Autodesk Inventor part; units mm, degrees
ref_plane "YZ Plane" through (0, 0, 0) normal (1, 0, 0) x (0, 1, 0)
ref_plane "XZ Plane" through (0, 0, 0) normal (0, 1, 0) x (-1, 0, 0)
ref_plane "XY Plane" through (0, 0, 0) normal (0, 0, 1) x (1, 0, 0)
sketch "Skizze1" plane through (0, 0, 0) normal (0, 0, 1) x (1, 0, 0)
  line L0 (-6.5297, -2.8796) -> (43.4703, -2.8796)
  line L1 (43.4703, -2.8796) -> (43.4703, 8.1204)
  line L2 (43.4703, 8.1204) -> (-6.5297, 8.1204)
  line L3 (-6.5297, 8.1204) -> (-6.5297, -2.8796)
  point P0 (0, 0)
  dimension "d0" = 50
  dimension "d1" = 11
extrude "Extrusion1" add sketch "Skizze1" along normal blind 7
sketch "Skizze2" plane through (-6.5297, 8.1204, 0) normal (0, 1, 0) x (1, 0, 0)
  line L0 (29.65, -5.55) -> (20.35, -5.55)
  line L1 (20.35, -5.55) -> (20.35, -1.45)
  line L2 (20.35, -1.45) -> (29.65, -1.45)
  line L3 (29.65, -1.45) -> (29.65, -5.55)
  line L4 (50, -7) -> (0, -7)
  line L5 (50, 0) -> (50, -7)
  line L6 (0, 0) -> (0, -7)
  point P0 (6.5297, 0)
  dimension "d4" = 9.3
  dimension "d5" = 4.1
  dimension "d6" = 1.45
  dimension "d7" = 20.35
  dimension "d8" = 20.35
extrude "Extrusion2" cut sketch "Skizze2" against normal blind 8.35
sketch "Skizze3" plane through (0, 0, 7) normal (0, 0, 1) x (1, 0, 0)
  line L0 (-6.5297, 8.1204) -> (-6.5297, -2.8796)
  line L1 (43.4703, 8.1204) -> (-6.5297, 8.1204)
  point P0 (0, 0)
  point P1 (5.9703, 2.2704)
  point P2 (18.4703, 2.2704)
  point P3 (30.9703, 2.2704)
  dimension "d11" = 12.5
  dimension "d12" = 12.5
  dimension "d13" = 12.5
  dimension "d14" = 5.85
hole "Bohrung1" at (5.9703, 2.2704, 7) at (18.4703, 2.2704, 7) at (30.9703, 2.2704, 7) direction (0, 0, -1) diameter 6.15 end through all
sketch "Skizze4" plane through (-6.5297, 8.1204, 0) normal (0, 1, 0) x (1, 0, 0)
  point P0 (6.5297, 0)
sketch "Skizze5" plane through (-6.5297, 8.1204, 0) normal (0, 1, 0) x (1, 0, 0)
  line L0 (50, 0) -> (0, 0)
  line L1 (0, 0) -> (0, -53.0037)
  line L2 (0, -53) -> (50, -53)
  line L3 (50, -53) -> (50, 46)
  line L4 (50, 46) -> (0, 46)
  line L5 (0, 46) -> (0, -53)
  point P0 (6.5297, 0)
  dimension "d22" = 50
  dimension "d23" = 99
  dimension "d24" = 46
extrude "Extrusion3" add sketch "Skizze5" along normal blind 3.5
sketch "Skizze6" plane through (-6.5297, 11.6204, 0) normal (0, 1, 0) x (1, 0, 0)
  line L0 (29.65, -1.45) -> (29.65, -5.55)
  line L1 (29.65, -1.45) -> (20.35, -1.45)
  line L2 (20.35, -1.45) -> (20.35, -5.55)
  line L3 (20.35, -5.55) -> (29.65, -5.55)
  line L4 (29.65, -5.55) -> (29.65, -1.45)
  point P0 (6.5297, 0)
extrude "Extrusion4" cut sketch "Skizze6" against normal blind 3.5
sketch "Skizze7" plane through (-6.5297, 11.6204, 0) normal (0, 1, 0) x (1, 0, 0)
  line L0 (0, -53) -> (50, -53)
  line L1 (50, -53) -> (42.5, -53)
  line L2 (42.5, -53) -> (42.5, -42.5)
  line L3 (42.5, -42.5) -> (50, -42.5)
  line L4 (50, -42.5) -> (50, -53)
  line L5 (0, -53) -> (7.5, -53)
  line L6 (7.5, -53) -> (7.5, -42.5)
  line L7 (7.5, -42.5) -> (0, -42.5)
  line L8 (0, -42.5) -> (0, -53)
  line L9 (0, 46) -> (0, -53)
  line L10 (0, 46) -> (7.5, 46)
  line L11 (7.5, 46) -> (7.5, 35.5)
  line L12 (7.5, 35.5) -> (0, 35.5)
  line L13 (0, 35.5) -> (0, 46)
  line L14 (50, -53) -> (50, 46)
  line L15 (50, 46) -> (42.5, 46)
  line L16 (42.5, 46) -> (42.5, 35.5)
  line L17 (42.5, 35.5) -> (50, 35.5)
  line L18 (50, 35.5) -> (50, 46)
  point P0 (6.5297, 0)
  dimension "d29" = 7.5
  dimension "d30" = 10.5
  dimension "d31" = 7.5
  dimension "d32" = 10.5
  dimension "d33" = 7.5
  dimension "d34" = 10.5
  dimension "d35" = 7.5
  dimension "d36" = 10.5
extrude "Extrusion5" add sketch "Skizze7" along normal blind 25
sketch "Skizze8" plane through (0.9703, 11.6204, -35.5) normal (1, 0, 0) x (0, 0, -1)
  point P0 (-35.5, -11.6204)
sketch "Skizze9" plane through (-6.5297, 36.6204, 0) normal (0, 1, 0) x (1, 0, 0)
  line L0 (50, -42.5) -> (50, 35.5)
  line L1 (0, 46) -> (50, 46)
  line L2 (50, 46) -> (50, 35.5)
  line L3 (50, 35.5) -> (0, 35.5)
  line L4 (0, 35.5) -> (0, 46)
  line L5 (50, -53) -> (50, -7)
  line L6 (0, -42.5) -> (50, -42.5)
  line L7 (50, -42.5) -> (50, -53)
  line L8 (50, -53) -> (0, -53)
  line L9 (0, -53) -> (0, -42.5)
  line L10 (50, -42.5) -> (42.5, -42.5)
  point P0 (6.5297, 0)
  dimension "d75" = 0
extrude "Extrusion6" add sketch "Skizze9" along normal blind 5
sketch "Skizze10" plane through (-6.5297, 41.6204, 0) normal (0, 1, 0) x (1, 0, 0)
  line L0 (50, 46) -> (0, 46)
  line L1 (0, -53) -> (50, -53)
  line L2 (42.5, -42.5) -> (42.5, -53)
  line L3 (42.5, 46) -> (42.5, 35.5)
  line L4 (7.5, 35.5) -> (7.5, 46)
  line L5 (7.5, -53) -> (7.5, -42.5)
  point P0 (6.5297, 0)
  point P1 (15.7518, 40.75)
  point P2 (25, 39.25)
  point P3 (33.5, 40.75)
  point P4 (15.6745, -47.75)
  point P5 (25, -46.5)
  point P6 (33.5, -47.75)
  dimension "d41" = 5.25
  dimension "d42" = 6.75
  dimension "d43" = 5.25
  dimension "d44" = 5.25
  dimension "d45" = 6.5
  dimension "d46" = 5.25
  dimension "d47" = 9
  dimension "d50" = 9
  dimension "d76" = 17.5
  dimension "d77" = 17.5
hole "Bohrung2" at (18.4703, 41.6204, 46.5) at (18.4703, 41.6204, -39.25) direction (0, -1, 0) diameter 6.15 depth 10 tip angle 118
sketch "Skizze11" plane through (-6.5297, 41.6204, 0) normal (0, 1, 0) x (1, 0, 0)
  line L0 (7.5, -53) -> (7.5, -42.5)
  line L1 (42.5, -42.5) -> (42.5, -53)
  line L2 (50, -42.5) -> (0, -42.5)
  line L3 (50, 46) -> (0, 46)
  line L4 (42.5, 46) -> (42.5, 35.5)
  line L5 (7.5, 35.5) -> (7.5, 46)
  point P0 (6.5297, 0)
  point P1 (16.5, -46.25)
  point P2 (33.5, -46.25)
  point P3 (16.5, 39.25)
  point P4 (33.5, 39.25)
  dimension "d60" = 9
  dimension "d61" = 9
  dimension "d62" = 3.75
  dimension "d63" = 3.75
  dimension "d64" = 6.75
  dimension "d65" = 6.75
  dimension "d66" = 9
  dimension "d67" = 9
hole "Bohrung3" at (9.9703, 41.6204, 46.25) at (26.9703, 41.6204, 46.25) at (9.9703, 41.6204, -39.25) at (26.9703, 41.6204, -39.25) direction (0, -1, 0) diameter 6.15 depth 31.5 tip angle 118
sketch "Skizze12" plane through (-6.5297, -2.8796, 0) normal (0, -1, 0) x (1, 0, 0)
  point P0 (6.5297, 0)
properties part number "Objektträgerhalter 1 fertig"
Can you work these out from the model? Positions are in its coordinate system, mm. A direction names the side the tool comes from. Round coordinates to 2 decimals unless told otherwise and drop trailing zeros. Loops run counter-clockwise (first coordinate to the right, second up) from the corner with the lowest first, then second, coordinate; pieces in that order, holes last. Notation, with made-up numbers: (10, -39) - (31, -39) arc R3 ccw to (31, -34) - close; hole circle Ø3 at (-7.5, 73.5). An arc over 180 degrees is marked (long way). Answer in a Markdown table with one row per item. Add a question column.
Q1. I need wall thicknesses on L1, parallel to X at y = 40, z = 46.5; L2, parallel to Z at x = 19.5, y = 11; L3, parallel to Z at x = 0, y = 18. Which ranges of each line are inside material? Lowest first, please.
Q2. For pin 1 Ø5.5 at (x, y) = (21, 4.5) entering from +Z; pin 2 Ø10 at (x, z) = (26.97, -39.25) entering from -Y; pin 3 Ø3.5 at (x, z) = (9.97, -39.25) entering from +Y, each with a flat end and sliding along its axis, tell me the tip position at first contact or that it passes through.
Q3. We'd pull the mould along X, two halves only. Please class faces 6 (the flat face through (18, 8.12, -23)), 7 (the flat face through (-6.53, 11, 3)), 8 (the cylindrical face through (9.047, 10.86, 49.183)): pulls with the +X half, pulls with the -X half, needs draft (parallel to the pull), parting line crosses it, or undercut.
Q4. I want a section at B-B on z = -28.5. List the corners of the cut face in (x, y) for me, and give its area (3 significant figures).
Q5. I want a section at A-A on y = 27. List the corners of the cut face in (x, z) for me, and give its area (3 significant figures).
Q6. Which directions (+Z, -Z, +X, -X, +Y, -Y) give clear straight access to the entire face, cutting with the end or side of a thin tool? Please do faces 1 (the flat face through (18, 6, 7)), 2 (the flat face through (23.12, 6, 3)), 3 (the flat face through (0.97, 24, 48)), 4 (the flat face through (18, 41.62, 50)), 5 (the flat face through (18, 40, 53)).
A:
| question | item | result |
|---|---|---|
| 1 | L1 | -6.53 to 6.91, 13.04 to 15.4, 21.55 to 23.91, 30.04 to 43.47 |
| 1 | L2 | -46 to 1.45, 5.55 to 53 |
| 1 | L3 | -46 to -35.5, 42.5 to 53 |
| 2 | pin 1 | z = 7 |
| 2 | pin 2 | y = 8.12 |
| 2 | pin 3 | y = 9.32 |
| 3 | face 6 | needs draft |
| 3 | face 7 | pulls with the -X half |
| 3 | face 8 | undercut |
| 4 | outline | (-6.53, 8.12) - (43.47, 8.12) - (43.47, 11.62) - (-6.53, 11.62) - close |
| 4 | area | 175 mm^2 |
| 5 | outline | (-6.53, -46) - (0.97, -46) - (0.97, -35.5) - (-6.53, -35.5) - close; (-6.53, 42.5) - (0.97, 42.5) - (0.97, 53) - (-6.53, 53) - close; (35.97, -46) - (43.47, -46) - (43.47, -35.5) - (35.97, -35.5) - close; (35.97, 42.5) - (43.47, 42.5) - (43.47, 53) - (35.97, 53) - close |
| 5 | area | 315 mm^2 |
| 6 | face 1 | +Z, +X, -X, -Y |
| 6 | face 2 | +Y |
| 6 | face 3 | +Z, -Z |
| 6 | face 4 | +Z, -Z, +X, -X, +Y |
| 6 | face 5 | +Z, +X, -X, +Y, -Y |
